```python
from build123d import *

# Parameters (mm, degrees)
F0_R     = 1.5875
F0_R_2   = 10.16
F1_DEPTH = 6.858
F2_T     = 2.54


# Not quite as in the source:
# - a shell that OpenCascade refuses in one call is made with other operations: the cavity is built on its own and cut out


with BuildPart() as f1:
    # F0 (on Front) → F1 (new body)
    with BuildSketch(Plane.XZ):
        with BuildLine():
            Line((9.9187, 16.2687), (-9.9187, 16.2687))
            ThreePointArc((-9.9187, 16.2687), (-14.4088280605, 14.4088280605), (-16.2687, 9.9187))
            Line((-16.2687, 9.9187), (-16.2687, -9.9187))
            ThreePointArc((-16.2687, -9.9187), (-14.4088280605, -14.4088280605), (-9.9187, -16.2687))
            Line((-9.9187, -16.2687), (9.9187, -16.2687))
            ThreePointArc((9.9187, -16.2687), (14.4088280605, -14.4088280605), (16.2687, -9.9187))
            Line((16.2687, -9.9187), (16.2687, 9.9187))
            ThreePointArc((16.2687, 9.9187), (14.4088280605, 14.4088280605), (9.9187, 16.2687))
        make_face()
        with Locations((-11.303, -11.303)):
            Circle(F0_R, mode=Mode.SUBTRACT)
        with Locations((11.303, -11.303)):
            Circle(F0_R, mode=Mode.SUBTRACT)
        with Locations((-11.303, 11.303)):
            Circle(F0_R, mode=Mode.SUBTRACT)
        Circle(F0_R_2, mode=Mode.SUBTRACT)
        with Locations((11.303, 11.303)):
            Circle(F0_R, mode=Mode.SUBTRACT)
    extrude(amount=F1_DEPTH)

    # F2: shell of thickness 2.54, made by hand


with BuildPart() as f2_core1:
    # F2_t2: copy of F1
    add(f1.part)

    # the walls: a layer under each face that stays
    f2_faces = [f2_core1.faces().sort_by_distance(p)[0] for p in [
        (-14.4088280605, -3.429, 14.4088280605),
        (-14.4088280605, -3.429, -14.4088280605),
        (14.4088280605, -3.429, -14.4088280605),
        (14.4088280605, -3.429, 14.4088280605),
        (-12.8905, -3.429, -11.303),
        (9.7155, -3.429, -11.303),
        (-12.8905, -3.429, 11.303),
        (-10.16, -3.429, 0),
        (9.7155, -3.429, 11.303),
        (-10.8458, 0, 0),
        (-10.8458, -6.858, 0),
    ]]
    thicken(f2_faces, amount=-F2_T, mode=Mode.SUBTRACT)


with BuildPart() as f1_1:
    add(f1.part)

    # what is left inside the walls is the cavity
    f2_cavity = [f2_core1.part.solids().sort_by_distance(p)[0] for p in [
        (-4.95935, -4.2926, 14.316209),
        (13.339963, -4.2926, -3.306233),
        (-13.339963, -4.2926, -3.306233),
        (0, -2.5654, -14.316209),
    ]]
    add(f2_cavity, mode=Mode.SUBTRACT)


solid = f1_1.part
```
Geometry: final body of the model. Coordinates: model frame, mm. A direction names the side the tool comes from. Coordinates: 2 decimals unless noted, no trailing zeros. Order: outer loops, then holes, each group sorted by start corner. A loop starts at its lowest first (then second) coordinate and runs counter-clockwise, first axis right, second up. Notation, with made-up numbers: (59.25, -36) - (64.25, -36) arc R13 ccw to (64.25, -14) - close; hole circle Ø2 at (17.25, 83.25). An arc over 180 degrees is marked (long way). Return JSON: item names as keys, results as strings. Group by question number.
1. Cut plane A-A (z = 0). Output: boundary loops of the cut face in (x, y).
2. Cut plane B-B (x = 0). Output: boundary loops of the cut face in (y, z), plus the area to 3 significant figures.
3. Pin query (flat end, axial travel): pin 1 (1.2 mm diameter, centred on x = 15.5, y = -4, fed in from +Z); pin 2 (0.5 mm diameter, centred on x = 15.5, y = -3.5, fed in from -Z); pin 3 (0.5 mm diameter, centred on x = -16, y = -3.5, fed in from +Z). Return the tip coordinate at first contact, or that it passes through.
4. Set-up query: faces 1 (the face through (-7.5, -6.858, 7.5)), 2 (the face through (9.919, -3, -16)). Return all of +Z, -Z, +X, -X, +Y, -Y with unobstructed straight access to the full face (end or side cutting, diameter ignored); none if empty.
5. Cut plane C-C (y = -3.75). Count the separate pieces of the cut face and the enclosed holes in it, plus the area to 3 significant figures.
6. Pull-direction query (Z, two-part tool) for faces 3 (the face through (0, -6, -16.269)), 4 (the face through (0, -6, 16.269)), 5 (the face through (16.269, -1, 0)), 6 (the face through (-16, -3, 9.919)); classes: pulls with the +Z half, pulls with the -Z half, needs draft (parallel to the pull), parting line crosses it, or undercut.
7. Material intervals for line 1 along Z through (x, y) = (0, -2.5); line 2 along Y through (x, z) = (-13.5, -1); line 3 along Z through (x, y) = (-11.5, -5.75), sorted ascending. Write a range as [from, to].
Resolved:
{
 "1": {"outline": "(-16.27, -6.86) - (-10.16, -6.86) - (-10.16, 0) - (-16.27, 0) - (-16.27, -2.54) - (-12.7, -2.54) - (-12.7, -4.32) - (-16.27, -4.32) - close; (10.16, -6.86) - (16.27, -6.86) - (16.27, -4.32) - (12.7, -4.32) - (12.7, -2.54) - (16.27, -2.54) - (16.27, 0) - (10.16, 0) - close"},
 "2": {"outline": "(-6.86, -16.27) - (-4.32, -16.27) - (-4.32, -12.7) - (-2.54, -12.7) - (-2.54, -16.27) - (0, -16.27) - (0, -10.16) - (-6.86, -10.16) - close; (-6.86, 10.16) - (0, 10.16) - (0, 16.27) - (-2.54, 16.27) - (-2.54, 12.7) - (-4.32, 12.7) - (-4.32, 16.27) - (-6.86, 16.27) - close", "area": "71.1 mm²"},
 "3": {"pin 1": "stops at z = 13.86", "pin 2": "stops at z = -13.37", "pin 3": "stops at z = 12.43"},
 "4": {"face 1": "+Z, -Z, +X, -X, -Y", "face 2": "-Z"},
 "5": {"separate pieces": "1", "enclosed holes": "5", "area": "375 mm²"},
 "6": {"face 3": "pulls with the -Z half", "face 4": "pulls with the +Z half", "face 5": "needs draft", "face 6": "undercut"},
 "7": {"line 1": "z = [-16.27, -10.16], [10.16, 16.27]", "line 2": "y = [-6.86, -4.32], [-2.54, 0]", "line 3": "z = [-16.07, -12.88], [-9.73, 9.73], [12.88, 16.07]"}
}
